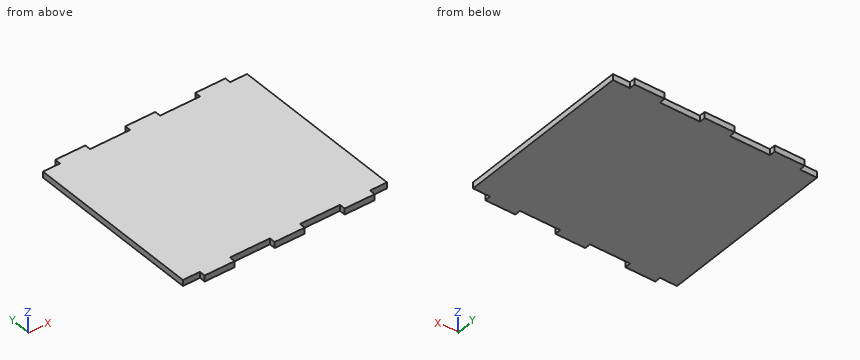
from build123d import *

# Parameters (mm, degrees)
SKETCH008_W                   = 102
SKETCH008_H                   = 95
PAD004_DEPTH                  = 3
SKETCH019_W                   = 8.5
SKETCH019_H                   = 3
SKETCH019_W_2                 = 20
POCKET014_DEPTH               = 281.841456
SKETCH019_MIRRORED017_2_W     = 8.5
SKETCH019_MIRRORED017_2_H     = 3
SKETCH019_MIRRORED017_2_W_2   = 20
POCKET014_MIRRORED017_2_DEPTH = 281.841456


with BuildPart() as part:
    # Sketch008 → Pad004 (new body)
    with BuildSketch(Plane.XY):
        Rectangle(SKETCH008_W, SKETCH008_H)
    extrude(amount=PAD004_DEPTH)

    # Sketch019 → Pocket014 (cut, through all)
    with BuildSketch(Plane.XY):
        with Locations((-46.75, 46)):
            Rectangle(SKETCH019_W, SKETCH019_H)
        with Locations((-17.5, 46)):
            Rectangle(SKETCH019_W_2, SKETCH019_H)
    pocket014 = extrude(amount=POCKET014_DEPTH, mode=Mode.SUBTRACT)

    # Sketch019 Mirrored017 2 → Pocket014 Mirrored017 2 (cut, through all)
    with BuildSketch(Plane(origin=(0, 0, 0), x_dir=(-1, 0, 0), z_dir=(0, 0, -1))):
        with Locations((-46.75, 46)):
            Rectangle(SKETCH019_MIRRORED017_2_W, SKETCH019_MIRRORED017_2_H)
        with Locations((-17.5, 46)):
            Rectangle(SKETCH019_MIRRORED017_2_W_2, SKETCH019_MIRRORED017_2_H)
    pocket014_mirrored017_2 = extrude(amount=-POCKET014_MIRRORED017_2_DEPTH, mode=Mode.SUBTRACT)

    # Mirrored018: Pocket014, Pocket014 Mirrored017 2 across Sketch019 H_Axis
    add(pocket014.mirror(Plane.ZX), mode=Mode.SUBTRACT)
    add(pocket014_mirrored017_2.mirror(Plane.ZX), mode=Mode.SUBTRACT)


with BuildPart() as part_1:
    # Body002 placement: moved
    add(part.part.moved(Location((0, 0, 2))))


solid = part_1.part
Source: CAD feature listing. Evaluate the final solid. Frame: model axes, mm. Round coordinates to 2 decimals unless told otherwise and drop trailing zeros. Loops run counter-clockwise (first coordinate to the right, second up) from the corner with the lowest first, then second, coordinate; pieces in that order, holes last. Notation, with made-up numbers: (51, 51) - (65, 51) arc R31 cw to (65, 78) - close; hole circle Ø10 at (71, 59). An arc over 180 degrees is marked (long way). Write item = value, one per line. Start each with the question number.
Item 1: Section query A-A on z = 4.15. Output: boundary loops of the cut face in (x, y).
Item 2: First-contact query: pin 1 Ø0.9 at (x, z) = (-48.5, 4) entering from +Y; pin 2 Ø0.9 at (y, z) = (46.5, 3) entering from -X; pin 3 Ø1.5 at (x, z) = (-46, 4) entering from -Y. Flat tips, straight axial feed; report the tip coordinate or a pass-through.
Item 3: Material intervals for line 1 (Y direction, x = -11.5, z = 3.55), sorted ascending.
Item 4: Section query B-B on x = -13.5. Output: boundary loops of the cut face in (y, z).
Results list:
q1.outline = (-51, -44.5) - (-42.5, -44.5) - (-42.5, -47.5) - (-27.5, -47.5) - (-27.5, -44.5) - (-7.5, -44.5) - (-7.5, -47.5) - (7.5, -47.5) - (7.5, -44.5) - (27.5, -44.5) - (27.5, -47.5) - (42.5, -47.5) - (42.5, -44.5) - (51, -44.5) - (51, 44.5) - (42.5, 44.5) - (42.5, 47.5) - (27.5, 47.5) - (27.5, 44.5) - (7.5, 44.5) - (7.5, 47.5) - (-7.5, 47.5) - (-7.5, 44.5) - (-27.5, 44.5) - (-27.5, 47.5) - (-42.5, 47.5) - (-42.5, 44.5) - (-51, 44.5) - close
q2.pin_1 = 44.5
q2.pin_2 = -42.5
q2.pin_3 = -44.5
q3.line_1 = -44.5 to 44.5
q4.outline = (-44.5, 2) - (44.5, 2) - (44.5, 5) - (-44.5, 5) - close
